```python
from build123d import *

# Parameters (mm, degrees)
CUT_EXTRUDE1_DEPTH      = 66.5
CUT_EXTRUDE1_DEPTH_BACK = 66.5


with BuildPart() as part:
    # Sketch1 → Revolve1 (revolve)
    with BuildSketch(Plane(origin=(0, 0, 0), x_dir=(0, 0, -1), z_dir=(1, 0, 0))):
        with BuildLine():
            Line((65.5, 0), (-65.5, 0))
            Line((-65.5, 0), (-65.5, 25))
            Line((-65.5, 25), (-49.5, 25))
            ThreePointArc((-49.5, 25), (-48.085786438, 25.585786438), (-47.5, 27))
            Line((-47.5, 27), (-47.5, 40))
            Line((-47.5, 40), (-19.5, 40))
            Line((-19.5, 40), (-17, 37.5))
            Line((-17, 37.5), (17, 37.5))
            Line((17, 37.5), (19.5, 40))
            Line((19.5, 40), (47.5, 40))
            Line((47.5, 40), (47.5, 27))
            ThreePointArc((47.5, 27), (48.085786438, 25.585786438), (49.5, 25))
            Line((49.5, 25), (65.5, 25))
            Line((65.5, 25), (65.5, 0))
        make_face()
    revolve(axis=Axis((0, 0, -65.5), (0, 0, 1)))

    # Sketch2 → Cut-Extrude1 (cut, two sides)
    with BuildSketch(Plane.XY) as cut_extrude1_sk:
        with BuildLine():
            Line((0, 40), (0, 13))
            Line((0, 13), (-12, 13))
            ThreePointArc((-12, 13), (-15, 10), (-12, 7))
            Line((-12, 7), (0, 7))
            Line((0, 7), (0, 0))
            Line((0, 0), (40, 0))
            ThreePointArc((40, 0), (28.284271247, 28.284271247), (0, 40))
        make_face()
    extrude(amount=CUT_EXTRUDE1_DEPTH, mode=Mode.SUBTRACT)
    extrude(cut_extrude1_sk.sketch, amount=-CUT_EXTRUDE1_DEPTH_BACK, mode=Mode.SUBTRACT)


solid = part.part
```
Check sheet for the modelled part. Datum: model origin and axes. Units: mm. A direction names the side the tool comes from. Give positions to 0.01 mm unless a question says otherwise; leave off trailing zeros. Order: outer loops, then holes, each group sorted by start corner. A loop starts at its lowest first (then second) coordinate and runs counter-clockwise, first axis right, second up. Notation, with made-up numbers: M 54.25,-2.5 L 82.25,-2.5 A32 ccw 82.25,29.5 Z; hole C 10.5,65 d7. An arc over 180 degrees is marked long. Answer in a Markdown table with one row per item.
1) Cross-section at A-A, the plane z = 56.5. Enter the section's corners in (x, y), plus the area to 3 significant figures.
Filled sheet:
| item | result |
|---|---|
| outline | M -12,7 A3 cw -12,13 L 0,13 L 0,25 A25 ccw long 25,0 L 0,0 L 0,7 Z |
| area | 1,390 mm2 |
2) Thickness scan on L1, parallel to Z at x = -34.5, y = 14.5; L2, parallel to Y at x = -12, z = -4; L3, parallel to Y at x = 1, z = -41. Record the ranges inside material, lowest first. Write a range as [from, to].
Filled sheet:
| item | result |
|---|---|
| L1 | z = [-47.5, 47.5] |
| L2 | y = [-35.53, 7], [13, 35.53] |
| L3 | y = [-39.99, 0] |
3) Gauge pin test, flat ends, axial feed: P1, Ø10, axis at x = -31.5, y = 16, coming from the -Z side; P2, Ø6, axis at x = -4, z = -9, coming from the -Y side; P3, Ø3, axis at y = 30, z = 27, coming from the -X side. Record the tip position at first contact, or that the pin passes through.
Filled sheet:
| item | result |
|---|---|
| P1 | stops at z = -47.5 |
| P2 | stops at y = -37.49 |
| P3 | stops at x = -28.07 |
4) Cross-section at B-B, the plane z = 10. Enter the section's corners in (x, y).
Filled sheet:
| item | result |
|---|---|
| outline | M -12,7 A3 cw -12,13 L 0,13 L 0,37.5 A37.5 ccw long 37.5,0 L 0,0 L 0,7 Z |
5) Access from +Z, -Z, +X, -X, +Y, -Y to the whole of each face (thin tool, end or side, straight path). Record for faces 5 (the conical face through (-27.491, -25.734, -17.156)), 6 (the cylindrical face through (-18.251, -17.085, 57.388)), 7 (the flat face through (-18, -21, -47.5)), 8 (the flat face through (20, 0, -1)).
Filled sheet:
| item | result |
|---|---|
| face 5 | none |
| face 6 | +Z |
| face 7 | -Z |
| face 8 | +Z, -Z, +X, +Y |
6) Release check for a two-part mould opening along Y. For faces 1 (the flat face through (-6, 13, -1)), 2 (the cylindrical face through (-15, 10, -1)), 3 (the flat face through (0, 27, -1)), 4 (the cylindrical face through (-18.251, -17.085, -57.612)) record: +Y half, -Y half, draft (parallel to the pull), parting line (faces both ways), or undercut.
Filled sheet:
| item | result |
|---|---|
| face 1 | undercut |
| face 2 | undercut |
| face 3 | draft |
| face 4 | parting line |
